Autodesk Inventor part; units mm, degrees
ref_plane "Start Plane" through (0, 0, 8.391) normal (0, 0, 1) x (1, 0, 0)
ref_plane "End Plane" through (0, 0, 60) normal (0, 0, 1) x (1, 0, 0)
ref_plane "Work Plane4" through (75, 8.6301, 8.6325) normal (0, -0.1736, -0.9848) x (1, 0, 0)
ref_plane "Start Plane" through (0, 0, 8.391) normal (0, 0, 1) x (1, 0, 0)
ref_plane "End Plane" through (0, 0, 60) normal (0, 0, 1) x (1, 0, 0)
sketch "Sketch" plane through (0, 0, 0) normal (0, 0, 1) x (1, 0, 0)
  line L0 (-10, -7) -> (-10, 7)
  line L1 (-7, 10) -> (7, 10)
  line L2 (10, 7) -> (10, -7)
  line L3 (7, -10) -> (-7, -10)
  arc A0 (-10, -7) -> (-7, -10) centre (-7, -7) ccw
  arc A1 (-7, 10) -> (-10, 7) centre (-7, 7) ccw
  arc A2 (10, 7) -> (7, 10) centre (7, 7) ccw
  arc A3 (7, -10) -> (10, -7) centre (7, -7) ccw
  arc A4 (-7, 8) -> (-8, 7) centre (-7, 7) ccw
  line L4 (-7, 8) -> (7, 8)
  arc A5 (8, 7) -> (7, 8) centre (7, 7) ccw
  line L5 (8, 7) -> (8, -7)
  arc A6 (7, -8) -> (8, -7) centre (7, -7) ccw
  line L6 (7, -8) -> (-7, -8)
  arc A7 (-8, -7) -> (-7, -8) centre (-7, -7) ccw
  line L7 (-8, -7) -> (-8, 7)
  line L8 (0, 14.8698) -> (0, -14.8698) construction
  line L9 (-14.8698, 0) -> (14.8698, 0) construction
  dimension "d7" = 3
  dimension "d10" = 20
  dimension "d11" = 20
  dimension "d12" = 2
  dimension "d15" = 10
  dimension "d16" = 10
extrude "Body" add sketch "Sketch" along normal up to surface (51.609 mm away) from surface at 8.391
sketch "Sketch3" plane through (0, 0, 0) normal (0, 0, 1) x (1, 0, 0)
  line L0 (0, 0) -> (10, 0)
ref_plane "Work Plane3" through (0, 0, 0) normal (0, -1, 0) x (1, 0, 0)
sketch "Sketch4" plane through (0, 0, 0) normal (0, -1, 0) x (1, 0, 0)
  line L0 (-2, 8.391) -> (12, 8.391)
  line L1 (-2, 60) -> (12, 60)
  dimension "d18" = 51.609
ref_plane "Work Plane4" through (75, 8.6301, 8.6325) normal (0, -0.1736, -0.9848) x (1, 0, 0)
split "Split1" plane through (75, 8.6301, 8.6325) removes the side toward (0, -0.1736, -0.9848)
ref_plane "Work Plane6" through (7.5, 49.6586, 233.7267) normal (0, 0.9318, -0.363) x (0, -0.363, -0.9318)
sketch "Sketch6" plane through (-7, -10, 60) normal (0, 0, 1) x (1, 0, 0)
  line L0 (14, 18) -> (0, 18)
  arc A0 (15, 17) -> (14, 18) centre (14, 17) ccw
  line L1 (15, 3) -> (15, 17)
  arc A1 (14, 2) -> (15, 3) centre (14, 3) ccw
  line L2 (0, 2) -> (14, 2)
  arc A2 (-1, 3) -> (0, 2) centre (0, 3) ccw
  line L3 (-1, 17) -> (-1, 3)
  arc A3 (0, 18) -> (-1, 17) centre (0, 17) ccw
  line L4 (-3, 3) -> (-3, 17)
  arc A4 (-3, 3) -> (0, 0) centre (0, 3) ccw
  line L5 (14, 0) -> (0, 0)
  arc A5 (14, 0) -> (17, 3) centre (14, 3) ccw
  line L6 (17, 17) -> (17, 3)
  arc A6 (17, 17) -> (14, 20) centre (14, 17) ccw
  line L7 (0, 20) -> (14, 20)
  arc A7 (0, 20) -> (-3, 17) centre (0, 17) ccw
  point P0 (7, 10)
extrude "Extrusion2" add sketch "Sketch6" along normal blind 153.26
split "Split3" plane through (7.5, 49.6586, 233.7267) removes the side toward (0, -0.9318, 0.363)
equation "\"d7\" = G_IR"
equation "\"d10\" = G_H"
equation "\"d11\" = G_W"
equation "\"d12\" = G_T"
equation "\"d15\" = 0.5 * d10"
equation "\"d16\" = 0.5 * d11"
equation "\"d3\" = G_L"
equation "\"G_W\" = 20"
equation "\"G_H\" = 20"
equation "\"G_T\" = 2"
equation "\"G_IR\" = 3"
equation "\"G_L\" = d18"
equation "\"G_OFFSET_START\" = -8.391"
equation "\"G_OFFSET_END\" = 0"
equation "\"d13\" = -G_OFFSET_START"
properties part number "ISO 12633-2 - 20x20x2 - 51,61" material "Steel, Mild"
The listing builds one solid part. Answer for the finished solid, in the listing's coordinates (mm). A direction names the side the tool comes from. Round coordinates to 2 decimals unless told otherwise and drop trailing zeros. Order: outer loops, then holes, each group sorted by start corner. A loop starts at its lowest first (then second) coordinate and runs counter-clockwise, first axis right, second up. Notation, with made-up numbers: (-15.5, -38.75) -> (12.5, -38.75) arc R29 cw to (12.5, -15.75) -> close; hole circle Ø6 at (19, 19.25). An arc over 180 degrees is marked (long way). One line per item, written item: value.
Item 1: For a pull along Y with two mould halves and no side action, classify faces 1 (the flat face through (8, 0, 53)), 2 (the flat face through (10, 0, 53)), 3 (the flat face through (8.75, 0.14, 10.13)), 4 (the flat face through (0, 8, 67)) as released by +Y, released by -Y, zero draft, split by the parting line, or undercut.
Taken from the geometry:
face 1: undercut
face 2: zero draft
face 3: released by -Y
face 4: undercut
Item 2: Find section B-B, the plane z = 56.5. Give the vertices of the cut face in (x, y), then the cut area to 3 significant figures.
Taken from the geometry:
outline: (-10, -7) arc R3 ccw to (-7, -10) -> (7, -10) arc R3 ccw to (10, -7) -> (10, 7) arc R3 ccw to (7, 10) -> (-7, 10) arc R3 ccw to (-10, 7) -> close; hole (-8, -7) arc R1 ccw to (-7, -8) -> (7, -8) arc R1 ccw to (8, -7) -> (8, 7) arc R1 ccw to (7, 8) -> (-7, 8) arc R1 ccw to (-8, 7) -> close
area: 137 mm2
Item 3: Find section C-C, the plane y = -4.75. Give the vertices of the cut face in (x, z), then the cut area to 3 significant figures.
Taken from the geometry:
outline: (-10, 10.99) -> (-8, 10.99) -> (-8, 94.06) -> (-10, 94.06) -> close; (8, 10.99) -> (10, 10.99) -> (10, 94.06) -> (8, 94.06) -> close
area: 332 mm2
Item 4: Straight lines are drawn through the part: L1, parallel to X at y = -2.25, z = 14; L2, parallel to Y at x = -6, z = 112. For each, find the intervals that lie inside material, in ascending order.
Taken from the geometry:
L1: x = -10 to -8, 8 to 10
L2: y = 8 to 10
Item 5: Find section D-D, the plane z = 93.5. Give the vertices of the cut face in (x, y), then the cut area to 3 significant figures.
Taken from the geometry:
outline: (-10, -4.97) -> (-8, -4.97) -> (-8, 7) arc R1 cw to (-7, 8) -> (7, 8) arc R1 cw to (8, 7) -> (8, -4.97) -> (10, -4.97) -> (10, 7) arc R3 ccw to (7, 10) -> (-7, 10) arc R3 ccw to (-10, 7) -> close
area: 88.4 mm2
Item 6: For faces 5 (the flat face through (0, -8, 48)), 6 (the cylindrical face through (-9.14, 9.1, 69.29)), determine the directions among +Z, -Z, +X, -X, +Y, -Y from which every point of the face is accessible in a straight line to the end or side of a thin tool.
Taken from the geometry:
face 5: +Z, -Z
face 6: +Z, -Z, -X, +Y
